from build123d import *

# Parameters (mm, degrees)
EXTRUDE_1_DEPTH     = 40
SKETCH_2_R          = 3
CUT_EXTRUDE_1_DEPTH = 10
SKETCH_3_R          = 3
CUT_EXTRUDE_2_DEPTH = 10


with BuildPart() as part:
    # Эскиз1 → Вытянуть-Тонкостенный1 (new body)
    with BuildSketch(Plane(origin=(0, 0, 0), x_dir=(0, 0, -1), z_dir=(1, 0, 0))):
        Polygon((25, 0), (0, 0), (0, 25), (3, 25), (3, 3), (25, 3), align=None)
    extrude(amount=EXTRUDE_1_DEPTH)

    # Эскиз2 → Вырез-Вытянуть1 (cut)
    with BuildSketch(Plane.XZ):
        with Locations((10, -14)):
            Circle(SKETCH_2_R)
        with Locations((30, -14)):
            Circle(SKETCH_2_R)
    extrude(amount=-CUT_EXTRUDE_1_DEPTH, mode=Mode.SUBTRACT)

    # Эскиз3 → Вырез-Вытянуть2 (cut)
    with BuildSketch(Plane.XY):
        with Locations((10, 14)):
            Circle(SKETCH_3_R)
        with Locations((30, 14)):
            Circle(SKETCH_3_R)
    extrude(amount=-CUT_EXTRUDE_2_DEPTH, mode=Mode.SUBTRACT)


solid = part.part
Verification items for the finished model (mm, model axes). A direction names the side the tool comes from. Coordinates: 2 decimals unless noted, no trailing zeros. Write each loop counter-clockwise with the first axis right and the second up, starting at its lowest first coordinate (ties: lowest second). Pieces come first, ordered by that corner, then holes. Notation, with made-up numbers: M 75,18 L 118,18 A32 ccw 118,52 Z; hole C 46.25,-30 d3. An arc over 180 degrees is marked long. One line per question, with ' | ' between items.
1) Material ranges on L1, parallel to Z at x = 10, y = 1.5; L2, parallel to Y at x = 30, z = -1.7; L3, parallel to Y at x = 35, z = -15, recorded low to high.
Solutions:
L1: -25 to -17, -11 to 0 | L2: 0 to 11, 17 to 25 | L3: 0 to 3
2) Sectioned sample at A-A on z = -14. Record the cut outline in (x, y), then the cut area to 3 significant figures.
Solutions:
outline: M 0,0 L 7,0 L 7,3 L 0,3 Z; M 13,0 L 27,0 L 27,3 L 13,3 Z; M 33,0 L 40,0 L 40,3 L 33,3 Z | area: 84.0 mm^2
3) Depth check by flat-ended pin: pin 1 Ø11 at (x, y) = (15.5, 12) entering from -Z; pin 2 Ø5.5 at (x, y) = (10, 14) entering from +Z; pin 3 Ø2 at (x, z) = (25, -12) entering from +Y. Enter the tip coordinate at first touch or a pass-through.
Solutions:
pin 1: z = -3 | pin 2: through | pin 3: y = 3
4) Sectioned sample at D-D on x = 19.5. Record the cut outline in (y, z), then the cut area to 3 significant figures.
Solutions:
outline: M 0,-25 L 3,-25 L 3,-3 L 25,-3 L 25,0 L 0,0 Z | area: 141 mm^2
5) Sectioned sample at C-C on x = 10. Record the cut outline in (y, z).
Solutions:
outline: M 0,-25 L 3,-25 L 3,-17 L 0,-17 Z; M 0,-11 L 3,-11 L 3,-3 L 11,-3 L 11,0 L 0,0 Z; M 17,-3 L 25,-3 L 25,0 L 17,0 Z
6) Access from +Z, -Z, +X, -X, +Y, -Y to the whole of each face (thin tool, end or side, straight path). Record for faces 5 (the face through (0, 2, -7)), 6 (the face through (20, 3, -14)).
Solutions:
face 5: +Z, -Z, -X, +Y, -Y | face 6: -Z, +X, -X, +Y
7) Release check for a two-part mould opening along Y. For faces 1 (the face through (20, 0, -13)), 2 (the face through (20, 14, -3)), 3 (the face through (27.6, 12.2, -1.5)), 4 (the face through (20, 25, -1)) record: +Y half, -Y half, draft (parallel to the pull), parting line (faces both ways), or undercut.
Solutions:
face 1: -Y half | face 2: draft | face 3: undercut | face 4: +Y half
8) Sectioned sample at B-B on y = 14. Record the cut outline in (x, z).
Solutions:
outline: M 0,-3 L 7,-3 L 7,0 L 0,0 Z; M 13,-3 L 27,-3 L 27,0 L 13,0 Z; M 33,-3 L 40,-3 L 40,0 L 33,0 Z
